Read the model definition and answer for the solid it produces. Units are mm, in the model's axes. Face numbers are marked on the shaded views. Give positions to 0.01 mm unless a question says otherwise; leave off trailing zeros. Order: outer loops, then holes, each group sorted by start corner. A loop starts at its lowest first (then second) coordinate and runs counter-clockwise, first axis right, second up. Notation, with made-up numbers: (76.5, -2) - (97.5, -2) arc R34 ccw to (97.5, 30) - close; hole circle Ø7 at (84, 6.25). An arc over 180 degrees is marked (long way). Use a Markdown table: item, result. Add a question column.
1. A cutting plane is placed at C-C on y = -27. Determine the outline of the cut face in (x, z), and give its area (3 significant figures).
2. A cutting plane is placed at B-B on x = 0. Determine the outline of the cut face in (y, z), and give its area (3 significant figures).
3. Consider L1, parallel to Y at x = 16, z = -1; L2, parallel to Z at x = 33, y = -32; L3, parallel to X at y = -17, z = 37.5. Determine where each line is inside the solid, lowest interval first.
4. Flat-ended cylindrical pins translate along their axes: P1, Ø5, axis at y = -13, z = -28, coming from the +X side; P2, Ø6, axis at x = 34.5, y = -22, coming from the +Z side; P3, Ø1, axis at y = -22.5, z = 23.5, coming from the +X side. Find the tip coordinate at first contact, or state that the pin passes through.
5. For a pull along X with two mould halves and no side action, classify the marked faces 1, 2 and 3 as released by +X, released by -X, zero draft, split by the parting line, or undercut.
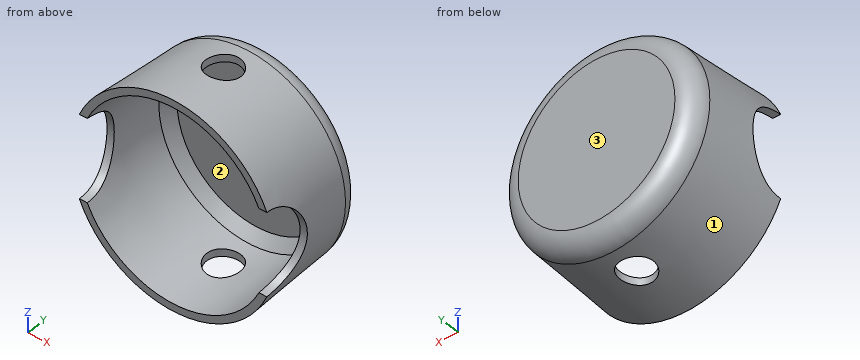
```python
from build123d import *

# Parameters (mm, degrees)
F0_R          = 50.8
F1_DEPTH      = 55.88
F1_TAPER      = -3
F2_T          = -3.81
F4_R          = 21.44690309
F5_DEPTH      = 58.166
F5_DEPTH_BACK = 65.786
F6_R          = 10.16
F7_SIZE       = 5.08
F9_R          = 8.89
F10_DEPTH     = 133.858


with BuildPart() as f1:
    # F0 (on Front) → F1 (new body)
    with BuildSketch(Plane.XZ):
        Circle(F0_R)
    extrude(amount=F1_DEPTH, taper=F1_TAPER)

    # F2
    f2_openings = [f1.faces().sort_by_distance(p)[0] for p in [
        (0, -55.88, 0),
    ]]
    offset(amount=F2_T, openings=f2_openings, kind=Kind.INTERSECTION)

    # F4 (on Right) → F5 (cut, two sides)
    with BuildSketch(Plane.YZ) as f5_sk:
        with Locations((-56.2342293561, 0)):
            Circle(F4_R)
    extrude(amount=-F5_DEPTH, mode=Mode.SUBTRACT)
    extrude(f5_sk.sketch, amount=F5_DEPTH_BACK, mode=Mode.SUBTRACT)

    # F6
    f6_edges = [f1.edges().sort_by_distance(p)[0] for p in [
        (-50.8, 0, 0),
    ]]
    fillet(f6_edges, radius=F6_R)

    # F7
    f7_edges = [f1.edges().sort_by_distance(p)[0] for p in [
        (-47.184445, -3.81, 0),
    ]]
    chamfer(f7_edges, length=F7_SIZE)

    # F9 (on offset) → F10 (cut)
    with BuildSketch(Plane.XY.offset(-64.008)):
        with Locations((0, -24.771042074)):
            Circle(F9_R)
    extrude(amount=F10_DEPTH, mode=Mode.SUBTRACT)


solid = f1.part
```
Output values:
| question | item | result |
|---|---|---|
| 1 | outline | (-8.61, -51.5) - (-8.61, -47.63) arc R48.4 cw to (-8.61, 47.63) - (-8.61, 51.5) arc R52.22 ccw to start; (8.61, -51.5) arc R52.22 ccw to (8.61, 51.5) - (8.61, 47.63) arc R48.4 cw to (8.61, -47.63) - close |
| 1 | area | 1,070 mm² |
| 2 | outline | (-55.88, -53.73) - (-33.66, -52.56) - (-33.66, -48.75) - (-55.88, -49.91) - close; (-55.88, 49.91) - (-33.66, 48.75) - (-33.66, 52.56) - (-55.88, 53.73) - close; (-15.88, -51.63) - (-9.63, -51.3) arc R10.16 ccw to (0, -41.16) - (0, 41.16) arc R10.16 ccw to (-9.63, 51.3) - (-15.88, 51.63) - (-15.88, 47.82) - (-8.88, 47.45) - (-3.81, 42.1) - (-3.81, -42.1) - (-8.88, -47.45) - (-15.88, -47.82) - close |
| 2 | area | 636 mm² |
| 3 | L1 | -3.81 to 0 |
| 3 | L2 | -40.8 to -35.76, 35.76 to 40.8 |
| 3 | L3 | -35.58 to -29.76, 29.76 to 35.58 |
| 4 | P1 | x = 44.73 |
| 4 | P2 | z = 41.32 |
| 4 | P3 | x = 46.62 |
| 5 | face 1 | split by the parting line |
| 5 | face 2 | undercut |
| 5 | face 3 | zero draft |
